Input: part model. Units: mm. Frame: model coordinates. A direction names the side the tool comes from. Round coordinates to 2 decimals unless told otherwise and drop trailing zeros. Loops run counter-clockwise (first coordinate to the right, second up) from the corner with the lowest first, then second, coordinate; pieces in that order, holes last.
1) Access query for faces 1 (the face through (2, 0, 17)), 2 (the face through (-3, 0, 0)), 3 (the face through (-4.3, 16.3, 3)), 4 (the face through (-3, -18, 3)). Directions: +Z, -Z, +X, -X, +Y, -Y. A direction counts if a zero-diameter tool reaches every point of the face in a straight line with its end or side. Return the directions, or none.
2) Section D-D, the plane y = -15.8. Return loops of the section in (x, z), and give its area (3 significant figures).
3) First-contact query: pin 1 (5 mm diameter, centred on x = -8, z = 26.5, fed in from +Y); pin 2 (6 mm diameter, centred on x = -6, z = 26, fed in from -Y); pin 3 (6 mm diameter, centred on x = 3, y = -11, fed in from +Z). Flat tips, straight axial feed; report the tip coordinate or a pass-through.
4) Ray query, line 1 along Y through (x, z) = (-2.5, 1.8); line 2 along X through (y, z) = (-8, 17.5); line 3 along Y through (x, z) = (-7.8, 21). Return the intervals inside material, ascending.
5) Section B-B, the plane z = 8. Return loops of the section in (x, y), and give its area (3 significant figures).
6) Section C-C, the plane x = -2.5. Return loops of the section in (y, z), and give its area (3 significant figures).
7) Draft query along Y for faces 5 (the face through (-8, 12.5, 10)), 6 (the face through (-10, 0, 13)), 7 (the face through (-4, 15, 1)), 8 (the face through (3.521, 0.477, 18.852)). Return one class per face: pulls with the +Y half, pulls with the -Y half, needs draft (parallel to the pull), parting line crosses it, or undercut.
8) Section A-A, the plane y = 0. Return loops of the section in (x, z).
from build123d import *

# Parameters (mm, degrees)
SCHIZZO1_W                    = 15
SCHIZZO1_H                    = 40
ESTRUSIONE_ESTRUSIONE1_DEPTH  = 3
SCHIZZO2_W                    = 15
SCHIZZO2_H                    = 25
ESTRUSIONE_ESTRUSIONE2_DEPTH  = 3
ESTRUSIONE_ESTRUSIONE4_DEPTH  = 3
ESTRUSIONE_ESTRUSIONE5_START  = -3
ESTRUSIONE_ESTRUSIONE5_DEPTH  = 3
TAGLIO_ESTRUSIONE1_DEPTH      = 42.800119617
TAGLIO_ESTRUSIONE1_DEPTH_BACK = 42.800119617
SCHIZZO7_R                    = 2.2
SCHIZZO9_R                    = 1.7
TAGLIO_ESTRUSIONE2_DEPTH      = 7


with BuildPart() as part:
    # Schizzo1 → Estrusione-Estrusione1 (new body)
    with BuildSketch(Plane.XY):
        with Locations((-2.5, 0)):
            Rectangle(SCHIZZO1_W, SCHIZZO1_H)
    extrude(amount=ESTRUSIONE_ESTRUSIONE1_DEPTH)

    # Schizzo2 → Estrusione-Estrusione2 (add)
    with BuildSketch(Plane.XY.offset(3)):
        with Locations((-2.5, 0)):
            Rectangle(SCHIZZO2_W, SCHIZZO2_H)
    extrude(amount=ESTRUSIONE_ESTRUSIONE2_DEPTH)

    # Schizzo5 → Estrusione-Estrusione4 (add)
    with BuildSketch(Plane.ZY.offset(10)):
        with BuildLine():
            Line((6, 12.5), (21, 12.5))
            ThreePointArc((21, 12.5), (33.5, 0), (21, -12.5))
            Line((21, -12.5), (6, -12.5))
            Line((6, -12.5), (6, 12.5))
        make_face()
    extrude(amount=-ESTRUSIONE_ESTRUSIONE4_DEPTH)

    # Schizzo6 → Estrusione-Estrusione5 (add)
    with BuildSketch(Plane(origin=(5, 0, 0), x_dir=(0, 0, -1), z_dir=(1, 0, 0)).offset(ESTRUSIONE_ESTRUSIONE5_START)):
        with BuildLine():
            Line((-6, -12.5), (-6, 12.5))
            Line((-6, 12.5), (-21, 12.5))
            ThreePointArc((-21, 12.5), (-33.5, 0), (-21, -12.5))
            Line((-21, -12.5), (-6, -12.5))
        make_face()
    extrude(amount=ESTRUSIONE_ESTRUSIONE5_DEPTH)

    # Schizzo7 → Taglio-Estrusione1 (cut, two sides: drawn at the far end of the back side and taken through both)
    with BuildSketch(Plane.ZY.offset(10).offset(-TAGLIO_ESTRUSIONE1_DEPTH_BACK)):
        with Locations(Location((21, 0, 0), (0, 0, 270))):
            Circle(SCHIZZO7_R)
    extrude(amount=TAGLIO_ESTRUSIONE1_DEPTH + TAGLIO_ESTRUSIONE1_DEPTH_BACK, mode=Mode.SUBTRACT)

    # Schizzo9 → Taglio-Estrusione2 (cut)
    with BuildSketch(Plane(origin=(0, 0, 0), x_dir=(-1, 0, 0), z_dir=(0, 0, -1))):
        with Locations((2.5, 15.8)):
            Circle(SCHIZZO9_R)
        with Locations(Location((2.5, -15.8, 0), (0, 0, 180))):
            Circle(SCHIZZO9_R)
    extrude(amount=-TAGLIO_ESTRUSIONE2_DEPTH, mode=Mode.SUBTRACT)


solid = part.part
Final values:
1. face 1: +Z, +Y, -Y
1. face 2: -Z, +X, -X, +Y, -Y
1. face 3: +Z, +X, -X, +Y
1. face 4: +Z, +X, -X, -Y
2. outline: (-10, 0) - (-4.2, 0) - (-4.2, 3) - (-10, 3) - close; (-0.8, 0) - (5, 0) - (5, 3) - (-0.8, 3) - close
2. area: 34.8 mm2
3. pin 1: stops at y = 12.13
3. pin 2: stops at y = -12.31
3. pin 3: stops at z = 30.6
4. line 1: y = -20 to -17.5, -14.1 to 14.1, 17.5 to 20
4. line 2: x = -10 to -7, 2 to 5
4. line 3: y = -12.5 to -2.2, 2.2 to 12.5
5. outline: (-10, -12.5) - (-7, -12.5) - (-7, 12.5) - (-10, 12.5) - close; (2, -12.5) - (5, -12.5) - (5, 12.5) - (2, 12.5) - close
5. area: 150 mm2
6. outline: (-20, 0) - (-17.5, 0) - (-17.5, 3) - (-20, 3) - close; (-14.1, 0) - (14.1, 0) - (14.1, 3) - (12.5, 3) - (12.5, 6) - (-12.5, 6) - (-12.5, 3) - (-14.1, 3) - close; (17.5, 0) - (20, 0) - (20, 3) - (17.5, 3) - close
6. area: 175 mm2
7. face 5: pulls with the +Y half
7. face 6: needs draft
7. face 7: undercut
7. face 8: undercut
8. outline: (-10, 0) - (5, 0) - (5, 18.8) - (2, 18.8) - (2, 6) - (-7, 6) - (-7, 18.8) - (-10, 18.8) - close; (-10, 23.2) - (-7, 23.2) - (-7, 33.5) - (-10, 33.5) - close; (2, 23.2) - (5, 23.2) - (5, 33.5) - (2, 33.5) - close
